Design review of the part built by this model. Coordinates are the model's own, in mm. Face numbers are marked on the shaded views. A direction names the side the tool comes from. Give positions to 0.01 mm unless a question says otherwise; leave off trailing zeros. Order: outer loops, then holes, each group sorted by start corner. A loop starts at its lowest first (then second) coordinate and runs counter-clockwise, first axis right, second up. Notation, with made-up numbers: (24, -3.5) -> (69, -3.5) arc R34 ccw to (69, 35.5) -> close; hole circle Ø1 at (25, 27.5). An arc over 180 degrees is marked (long way). One line per item, written item: value. Start each with the question number.
1) Wall thickness on line 1 along Z through (x, y) = (24, 151.5); line 2 along X through (y, z) = (-42, 536); line 3 along Y through (x, z) = (-46.5, 368.5): over which ranges is each line inside the solid? List them lowest first. Write a range as from..to.
2) For pin 1 (6 mm diameter, centred on x = -20.5, z = 395, fed in from +Y); pin 2 (24 mm diameter, centred on x = -93, y = 25.5, fed in from -Z); pin 3 (9 mm diameter, centred on x = -96, y = 42.5, fed in from +Z), all flat-tipped, find the tip position at first contact; note any pin that passes through.
3) Consider section C-C (y = -26). State how many separate pieces and enclosed holes the cut face has, plus the area to 3 significant figures.
4) Consider section A-A (z = 658.5). State the section outline as (x, y) points.
5) Tool access review of the marked faces 1, 2, 3 and 4: name each direction out of +Z, -Z, +X, -X, +Y, -Y from which nothing blocks a thin tool from reaching the whole face with its end or side.
6) Consider section B-B (x = 18). State the section outline as (y, z) points, plus the area to 3 significant figures.
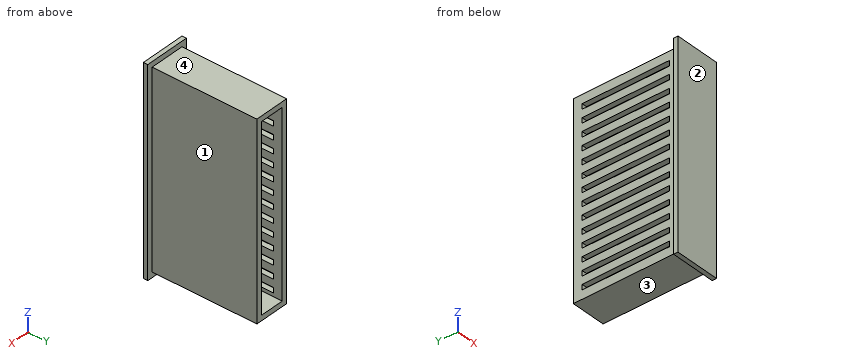
from build123d import *

# Parameters (mm, degrees)
F0_W     = 200
F0_H     = 600
F1_DEPTH = 1100
F2_W     = 140
F2_H     = 1040
F3_DEPTH = 600
F4_W     = 500
F4_H     = 30
F5_DEPTH = 30
F6_W     = 260
F6_H     = 1160
F6_W_2   = 200
F6_H_2   = 1100
F7_DEPTH = 25


with BuildPart() as f1:
    # F0 (on Top) → F1 (new body)
    with BuildSketch(Plane.XY):
        with Locations((-10.210905, -5.170632)):
            Rectangle(F0_W, F0_H)
    extrude(amount=F1_DEPTH)

    # F2 (on face) → F3 (cut, through all)
    with BuildSketch(Plane.XZ.offset(305.170632)):
        with Locations((-10.210905, 550)):
            Rectangle(F2_W, F2_H)
    extrude(amount=-F3_DEPTH, mode=Mode.SUBTRACT)

    # F4 (on face) → F5 (cut)
    with BuildSketch(Plane(origin=(-110.210905, 0, 0), x_dir=(0, -1, 0), z_dir=(-1, 0, 0))):
        with Locations((5.170632, 1035)):
            Rectangle(F4_W, F4_H)
        with Locations((5.170632, 960.4)):
            Rectangle(F4_W, F4_H)
        with Locations((5.170632, 885.8)):
            Rectangle(F4_W, F4_H)
        with Locations((5.170632, 811.2)):
            Rectangle(F4_W, F4_H)
        with Locations((5.170632, 736.6)):
            Rectangle(F4_W, F4_H)
        with Locations((5.170632, 662)):
            Rectangle(F4_W, F4_H)
        with Locations((5.170632, 587.4)):
            Rectangle(F4_W, F4_H)
        with Locations((5.170632, 512.8)):
            Rectangle(F4_W, F4_H)
        with Locations((5.170632, 438.2)):
            Rectangle(F4_W, F4_H)
        with Locations((5.170632, 363.6)):
            Rectangle(F4_W, F4_H)
        with Locations((5.170632, 289)):
            Rectangle(F4_W, F4_H)
        with Locations((5.170632, 214.4)):
            Rectangle(F4_W, F4_H)
        with Locations((5.170632, 139.8)):
            Rectangle(F4_W, F4_H)
        with Locations((5.170632, 65.2)):
            Rectangle(F4_W, F4_H)
    extrude(amount=-F5_DEPTH, mode=Mode.SUBTRACT)

    # F6 (on face) → F7 (join)
    with BuildSketch(Plane.XZ.offset(305.170632)):
        with Locations((-10.210905, 550)):
            Rectangle(F6_W, F6_H)
        with Locations((-10.210905, 550)):
            Rectangle(F6_W_2, F6_H_2, mode=Mode.SUBTRACT)
        with Locations((-10.210905, 550)):
            Rectangle(F6_W_2, F6_H_2)
    extrude(amount=F7_DEPTH)


solid = f1.part
Checked values:
1. line 1: z = 0..30, 1070..1100
1. line 2: x = -110.21..-80.21, 59.79..89.79
1. line 3: y = -330.17..-305.17
2. pin 1: stops at y = -305.17
2. pin 2: stops at z = 0
2. pin 3: stops at z = 1100
3. separate pieces: 14
3. enclosed holes: 0
3. area: 61,800 mm^2
4. outline: (-140.21, -330.17) -> (119.79, -330.17) -> (119.79, -305.17) -> (89.79, -305.17) -> (89.79, 294.83) -> (59.79, 294.83) -> (59.79, -305.17) -> (-80.21, -305.17) -> (-80.21, -255.17) -> (-110.21, -255.17) -> (-110.21, -305.17) -> (-140.21, -305.17) -> close; (-110.21, 244.83) -> (-80.21, 244.83) -> (-80.21, 294.83) -> (-110.21, 294.83) -> close
5. face 1: +Z, -Z, +X, +Y
5. face 2: +Z, -Z, +X, -X, -Y
5. face 3: -Z, +X, -X, +Y
5. face 4: +Z, +X, -X, +Y
6. outline: (-330.17, -30) -> (-305.17, -30) -> (-305.17, 0) -> (294.83, 0) -> (294.83, 30) -> (-305.17, 30) -> (-305.17, 1070) -> (294.83, 1070) -> (294.83, 1100) -> (-305.17, 1100) -> (-305.17, 1130) -> (-330.17, 1130) -> close
6. area: 65,000 mm^2
